Can you work these out from the model? Positions are in its coordinate system, mm. Coordinates: 2 decimals unless noted, no trailing zeros. Order: outer loops, then holes, each group sorted by start corner. A loop starts at its lowest first (then second) coordinate and runs counter-clockwise, first axis right, second up. Notation, with made-up numbers: (24.5, 54) -> (53.5, 54) arc R16 cw to (53.5, 73) -> close; hole circle Ø9 at (8, -3.75). An arc over 180 degrees is marked (long way). Answer in a Markdown table with one row per item.
```python
from build123d import *

# Parameters (mm, degrees)
F0_R     = 6
F1_DEPTH = 20


with BuildPart() as f1:
    # F0 (on Top) → F1 (new body)
    with BuildSketch(Plane.XY):
        with BuildLine():
            ThreePointArc((0, 6), (-4.242641, -4.242641), (6, 0))
            ThreePointArc((6, 0), (4.242641, 4.242641), (0, 6))
        make_face()
        with BuildLine():
            ThreePointArc((8.556611, 8.413347), (6, 25), (8.556611, 41.586653))
            ThreePointArc((8.556611, 41.586653), (0, 62), (-8.556611, 41.586653))
            ThreePointArc((-8.556611, 41.586653), (-6, 25), (-8.556611, 8.413347))
            ThreePointArc((-8.556611, 8.413347), (0, -12), (8.556611, 8.413347))
        make_face()
        with BuildLine():
            ThreePointArc((0, 6), (4.242641, 4.242641), (6, 0))
            ThreePointArc((6, 0), (-4.242641, -4.242641), (0, 6))
        make_face(mode=Mode.SUBTRACT)
        with Locations((0, 50)):
            Circle(F0_R, mode=Mode.SUBTRACT)
    extrude(amount=F1_DEPTH)


solid = f1.part
```
(1) Suppose I cut it at D-D (x = -10.25). Please give me the cut outline in (y, z).
Response values:
| item | result |
|---|---|
| outline | (-6.24, 0) -> (6.24, 0) -> (6.24, 20) -> (-6.24, 20) -> close; (43.76, 0) -> (56.24, 0) -> (56.24, 20) -> (43.76, 20) -> close |
(2) We'd pull the mould along X, two halves only. Please class faces 1 (the cylindrical face through (0, -12, 10)), 2 (the cylindrical face through (-1.301, 44.143, 9.86)), 3 (the flat face through (0, 26, 0)): +X half, -X half, draft (parallel to the pull), parting line (faces both ways), or undercut.
Response values:
| item | result |
|---|---|
| face 1 | parting line |
| face 2 | undercut |
| face 3 | draft |
(3) Suppose I cut it at C-C (x = 1.25). Please give me the cut outline in (y, z).
Response values:
| item | result |
|---|---|
| outline | (-11.93, 0) -> (-5.87, 0) -> (-5.87, 20) -> (-11.93, 20) -> close; (5.87, 0) -> (44.13, 0) -> (44.13, 20) -> (5.87, 20) -> close; (55.87, 0) -> (61.93, 0) -> (61.93, 20) -> (55.87, 20) -> close |
(4) Suppose I cut it at A-A (z = 7.5). Please give me the cut outline in (x, y).
Response values:
| item | result |
|---|---|
| outline | (-8.56, 8.41) arc R12 ccw (long way) to (8.56, 8.41) arc R55.08 cw to (8.56, 41.59) arc R12 ccw (long way) to (-8.56, 41.59) arc R55.08 cw to start; hole circle Ø12 at (0, 50); hole (0, 6) arc R6 ccw (long way) to (6, 0) arc R6 ccw to start |
(5) I need wall thicknesses on line 1 (Y direction, x = 0, z = 14.75); line 2 (Y direction, x = 4.75, z = 6.5); line 3 (X direction, y = 46.5, z = 16.5). Which ranges of each line are inside material? Lowest first, please. Write a range as [from, to].
Response values:
| item | result |
|---|---|
| line 1 | [-12, -6], [6, 44], [56, 62] |
| line 2 | [-11.02, -3.67], [3.67, 46.33], [53.67, 61.02] |
| line 3 | [-11.48, -4.87], [4.87, 11.48] |
(6) Suppose I cut it at B-B (y = 50). Please give me the cut outline in (x, z).
Response values:
| item | result |
|---|---|
| outline | (-12, 0) -> (-6, 0) -> (-6, 20) -> (-12, 20) -> close; (6, 0) -> (12, 0) -> (12, 20) -> (6, 20) -> close |
(7) Will these pins go through, and if not, where does the flat tip stop? pin 1 Ø7 at (x, y) = (0, 50) entering from -Z; pin 2 Ø1.5 at (y, z) = (27, 8.5) entering from -X; pin 3 Ø1 at (y, z) = (39.5, 2) entering from -X; pin 4 Ø1.5 at (y, z) = (-4, 12.5) entering from +X.
Response values:
| item | result |
|---|---|
| pin 1 | through |
| pin 2 | x = -6.07 |
| pin 3 | x = -8.08 |
| pin 4 | x = 11.55 |
